```python
from build123d import *

# Parameters (mm, degrees)
SKETCH1_R           = 1.5
BOSS_EXTRUDE1_DEPTH = 8
BOSS_EXTRUDE2_DEPTH = 30
FILLET1_R           = 2
BOSS_EXTRUDE3_DEPTH = 9
SKETCH4_R           = 11
BOSS_EXTRUDE4_DEPTH = 2
SKETCH5_R           = 2.5
BOSS_EXTRUDE5_DEPTH = 22
BOSS_EXTRUDE6_START = 10
SKETCH6_R           = 2.5
BOSS_EXTRUDE6_DEPTH = 10


with BuildPart() as part:
    # Sketch1 → Boss-Extrude1 (new body)
    with BuildSketch(Plane(origin=(0, 0, 0), x_dir=(1, 0, 0), z_dir=(0, 1, 0))):
        Polygon((-17, 21), (17, 21), (21, 17), (21, -17), (17, -21), (-17, -21), (-21, -17), (-21, 17), align=None)
        with Locations(Location((-15.5, 15.5, 0), (0, 0, 270))):
            Circle(SKETCH1_R, mode=Mode.SUBTRACT)
        with Locations(Location((-15.5, -15.5, 0), (0, 0, 270))):
            Circle(SKETCH1_R, mode=Mode.SUBTRACT)
        with Locations(Location((15.5, -15.5, 0), (0, 0, 270))):
            Circle(SKETCH1_R, mode=Mode.SUBTRACT)
        with Locations(Location((15.5, 15.5, 0), (0, 0, 270))):
            Circle(SKETCH1_R, mode=Mode.SUBTRACT)
    extrude(amount=BOSS_EXTRUDE1_DEPTH)

    # Sketch2 → Boss-Extrude2 (add)
    with BuildSketch(Plane.XZ):
        Polygon((-12.75, 20.75), (12.75, 20.75), (20.75, 12.75), (20.75, -12.75), (12.75, -20.75), (-12.75, -20.75), (-20.75, -12.75), (-20.75, 12.75), align=None)
    extrude(amount=BOSS_EXTRUDE2_DEPTH)

    # Fillet1
    fillet1_edges = [part.edges().sort_by_distance(p)[0] for p in [
        (20.75, -15, 12.75),
        (12.75, -15, 20.75),
        (-12.75, -15, 20.75),
        (-20.75, -15, 12.75),
        (-20.75, -15, -12.75),
        (-12.75, -15, -20.75),
        (12.75, -15, -20.75),
        (20.75, -15, -12.75),
    ]]
    fillet(fillet1_edges, radius=FILLET1_R)

    # Sketch3 → Boss-Extrude3 (add)
    with BuildSketch(Plane.XZ.offset(30)):
        Polygon((-21, 17), (-21, -17), (-17, -21), (17, -21), (21, -17), (21, 17), (17, 21), (-17, 21), align=None)
    extrude(amount=BOSS_EXTRUDE3_DEPTH)

    # Sketch4 → Boss-Extrude4 (add)
    with BuildSketch(Plane(origin=(0, 8, 0), x_dir=(1, 0, 0), z_dir=(0, 1, 0))):
        with Locations(Location((0, 0, 0), (0, 0, 90))):
            Circle(SKETCH4_R)
    extrude(amount=BOSS_EXTRUDE4_DEPTH)

    # Sketch5 → Boss-Extrude5 (add)
    with BuildSketch(Plane(origin=(0, 10, 0), x_dir=(1, 0, 0), z_dir=(0, 1, 0))):
        with Locations(Location((0, 0, 0), (0, 0, 270))):
            Circle(SKETCH5_R)
    extrude(amount=BOSS_EXTRUDE5_DEPTH)

    # Sketch6 → Boss-Extrude6 (add)
    with BuildSketch(Plane.XZ.offset(39).offset(BOSS_EXTRUDE6_START)):
        with Locations(Location((0, 0, 0), (0, 0, 90))):
            Circle(SKETCH6_R)
    extrude(amount=-BOSS_EXTRUDE6_DEPTH)


solid = part.part
```
Build history of the part. All positions in model axes, mm. A direction names the side the tool comes from. Coordinates: 2 decimals unless noted, no trailing zeros. Write each loop counter-clockwise with the first axis right and the second up, starting at its lowest first coordinate (ties: lowest second). Pieces come first, ordered by that corner, then holes.
1. 3-axis set-ups, long thin cutter, end or side, ignore diameter. For faces 1 (the cylindrical face through (2.44, -44.07, -0.54)), 2 (the flat face through (16.7, -14.8, 16.8)), 3 (the flat face through (-16.7, -14.8, -16.8)), 4 (the cylindrical face through (15.57, 3.94, 14)), 5 (the flat face through (-16.8, -14.8, 16.7)): which of +Z, -Z, +X, -X, +Y, -Y reach the whole face in a straight line?
Answer block:
face 1: -Y
face 2: +Z, +X
face 3: -Z, -X
face 4: +Y
face 5: +Z, -X
2. Pull direction X, two halves, no side cores. Call faces 6 (the flat face through (-15, 0, -15)), 7 (the flat face through (0, -34, 21)), 8 (the flat face through (16.8, -14.8, -16.7)): released by +X, released by -X, zero draft, split by the parting line, or undercut.
Answer block:
face 6: undercut
face 7: zero draft
face 8: released by +X
3. Band-saw the part on B-B, the plane z = 0. Give the cut face in (x, y), and give its area (3 significant figures).
Answer block:
outline: (-21, -39) - (-2.5, -39) - (-2.5, -49) - (2.5, -49) - (2.5, -39) - (21, -39) - (21, -30) - (20.75, -30) - (20.75, 0) - (21, 0) - (21, 8) - (11, 8) - (11, 10) - (2.5, 10) - (2.5, 32) - (-2.5, 32) - (-2.5, 10) - (-11, 10) - (-11, 8) - (-21, 8) - (-21, 0) - (-20.75, 0) - (-20.75, -30) - (-21, -30) - close
area: 2,160 mm2
4. Band-saw the part on D-D, the plane z = 15.5. Give the cut face in (x, y).
Answer block:
outline: (-21, -39) - (21, -39) - (21, -30) - (18, -30) - (18, 0) - (21, 0) - (21, 8) - (17, 8) - (17, 0) - (14, 0) - (14, 8) - (-14, 8) - (-14, 0) - (-17, 0) - (-17, 8) - (-21, 8) - (-21, 0) - (-18, 0) - (-18, -30) - (-21, -30) - close
5. Drop flat-ended pins along their axis: pin 1 (0.9 mm diameter, centred on x = 16, z = 15, fed in from +Y); pin 2 (5 mm diameter, centred on x = 15.5, z = 15.5, fed in from +Y); pin 3 (12 mm diameter, centred on y = 24, z = 3, fed in from +X). Give the stop position or say it passes through.
Answer block:
pin 1: stops at y = 0
pin 2: stops at y = 8
pin 3: stops at x = 2.5
6. Band-saw the part on A-A, the plane x = -15.5. Give the cut face in (y, z).
Answer block:
outline: (-39, -21) - (-30, -21) - (-30, -18) - (0, -18) - (0, -21) - (8, -21) - (8, -17) - (0, -17) - (0, -14) - (8, -14) - (8, 14) - (0, 14) - (0, 17) - (8, 17) - (8, 21) - (0, 21) - (0, 18) - (-30, 18) - (-30, 21) - (-39, 21) - close
7. Band-saw the part on C-C, the plane y = -24. Give the cut face in (x, z).
Answer block:
outline: (-20.75, -11.92) arc R2 ccw to (-20.16, -13.34) - (-13.34, -20.16) arc R2 ccw to (-11.92, -20.75) - (11.92, -20.75) arc R2 ccw to (13.34, -20.16) - (20.16, -13.34) arc R2 ccw to (20.75, -11.92) - (20.75, 11.92) arc R2 ccw to (20.16, 13.34) - (13.34, 20.16) arc R2 ccw to (11.92, 20.75) - (-11.92, 20.75) arc R2 ccw to (-13.34, 20.16) - (-20.16, 13.34) arc R2 ccw to (-20.75, 11.92) - close
8. Drill centre lines: probe 1 along X at (y, z) = (3.75, 15.5); probe 2 along Z at (x, y) = (-15, 3); probe 3 along Y at (x, z) = (-4, -19). Where is each one in solid material? Low to high.
Answer block:
probe 1: x = -21 to -17, -14 to 14, 17 to 21
probe 2: z = -21 to -16.91, -14.09 to 14.09, 16.91 to 21
probe 3: y = -39 to 8
